Verification items for the finished model (mm, model axes). Face numbers are marked on the shaded views. A direction names the side the tool comes from. Round coordinates to 2 decimals unless told otherwise and drop trailing zeros. Write each loop counter-clockwise with the first axis right and the second up, starting at its lowest first coordinate (ties: lowest second). Pieces come first, ordered by that corner, then holes. Notation, with made-up numbers: (64.25, 41) - (107.25, 41) arc R13 ccw to (107.25, 47) - close; hole circle Ø4 at (83, 71.5). An arc over 180 degrees is marked (long way). Answer as a JSON object with one key per item and string values.
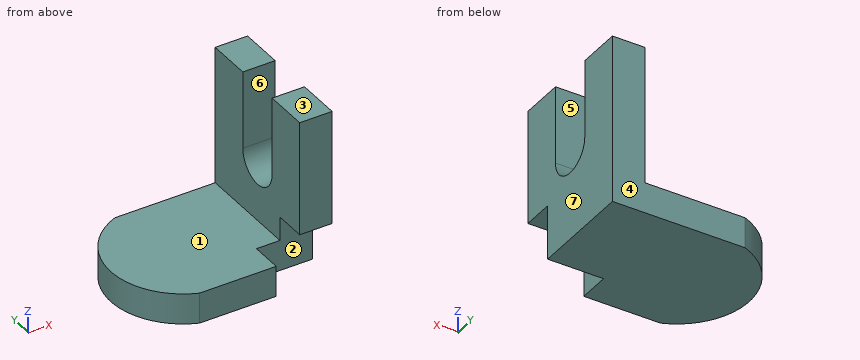
```python
from build123d import *

# Parameters (mm, degrees)
F0_W     = 13.8414949179
F0_H     = 57.7164180577
F1_DEPTH = 13.1
F2_DEPTH = 72.2
F4_DEPTH = 13.8424949179
F6_DEPTH = 13.5


with BuildPart() as f1:
    # F0 (on Top) → F1 (new body)
    with BuildSketch(Plane.XY):
        with Locations((21.4151442051, 0)):
            Rectangle(F0_W, F0_H)
        with BuildLine():
            Line((-28.335891664, -28.8582090288), (14.4943967462, -28.8582090288))
            Line((14.4943967462, -28.8582090288), (14.4943967462, 28.8582090288))
            Line((14.4943967462, 28.8582090288), (-28.335891664, 28.8582090288))
            ThreePointArc((-28.335891664, 28.8582090288), (-48.1865539217, 0), (-28.335891664, -28.8582090288))
        make_face()
    extrude(amount=F1_DEPTH)

    # F0 (on Top) → F2 (join)
    with BuildSketch(Plane.XY):
        with Locations((21.4151442051, 0)):
            Rectangle(F0_W, F0_H)
    extrude(amount=F2_DEPTH)

    # F3 (on face) → F4 (cut, through all)
    with BuildSketch(Plane(origin=(14.4943967462, 0, 0), x_dir=(0, -1, 0), z_dir=(-1, 0, 0))):
        with BuildLine():
            Line((10, 72.2), (-10, 72.2))
            Line((-10, 72.2), (-10, 38.9287173748))
            ThreePointArc((-10, 38.9287173748), (0, 28.9287173748), (10, 38.9287173748))
            Line((10, 38.9287173748), (10, 72.2))
        make_face()
        with BuildLine():
            ThreePointArc((10, 72.2), (0, 82.2), (-10, 72.2))
            Line((-10, 72.2), (10, 72.2))
        make_face()
    extrude(amount=-F4_DEPTH, mode=Mode.SUBTRACT)

    # F5 (on face) → F6 (cut)
    with BuildSketch(Plane.XZ.offset(28.8582090288)):
        Polygon((28.335891664, 23.2873037457), (14.4943967462, 23.2873037457), (14.4943967462, 13.1), (4.4452203438, 13.1), (4.4452203438, 0), (28.335891664, 0), align=None)
    extrude(amount=-F6_DEPTH, mode=Mode.SUBTRACT)


solid = f1.part
```
1. Mould release check, pull along Y, two halves, no side actions. Record for the marked faces 4, 5, 6 and 7: released by +Y, released by -Y, zero draft, split by the parting line, or undercut.
Completed:
{"face 4": "released by +Y", "face 5": "undercut", "face 6": "undercut", "face 7": "zero draft"}
2. Cross-section at C-C (x = -26.5). Record the boundary of the cut face in (y, z).
Completed:
{"outline": "(-28.86, 0) - (28.86, 0) - (28.86, 13.1) - (-28.86, 13.1) - close"}
3. Material ranges on probe 1 along Y at (x, z) = (15, 43); probe 2 along Z at (x, y) = (-1, -23.5); probe 3 along X at (y, z) = (-11.5, 18), recorded low to high. Write a range as from..to.
Completed:
{"probe 1": "y = -28.86..-10, 10..28.86", "probe 2": "z = 0..13.1", "probe 3": "x = 14.49..28.34"}
4. Cross-section at A-A (z = 58.5). Record the boundary of the cut face in (x, y), plus the area to 3 significant figures.
Completed:
{"outline": "(14.49, -28.86) - (28.34, -28.86) - (28.34, -10) - (14.49, -10) - close; (14.49, 10) - (28.34, 10) - (28.34, 28.86) - (14.49, 28.86) - close", "area": "522 mm^2"}
5. Go/stop test with flat-tipped pins: pin 1 (17.5 mm diameter, centred on x = -2, y = -6, fed in from +Z); pin 2 (4 mm diameter, centred on y = -8, z = 26.5, fed in from -X); pin 3 (7 mm diameter, centred on x = 23.5, y = -20.5, fed in from -Z). Record where each tip stops, or that it passes through.
Completed:
{"pin 1": "stops at z = 13.1", "pin 2": "stops at x = 14.49", "pin 3": "stops at z = 23.29"}
6. Cross-section at D-D (z = 27). Record the boundary of the cut face in (x, y).
Completed:
{"outline": "(14.49, -28.86) - (28.34, -28.86) - (28.34, 28.86) - (14.49, 28.86) - close"}
7. Access from +Z, -Z, +X, -X, +Y, -Y to the whole of each face (thin tool, end or side, straight path). Record for the marked faces 1, 2 and 3.
Completed:
{"face 1": "+Z, -X, +Y, -Y", "face 2": "-Z, +X, -Y", "face 3": "+Z, +X, -X, +Y, -Y"}
8. Cross-section at B-B (y = 0). Record the boundary of the cut face in (x, z).
Completed:
{"outline": "(-48.19, 0) - (28.34, 0) - (28.34, 28.93) - (14.49, 28.93) - (14.49, 13.1) - (-48.19, 13.1) - close"}
